Here's how the part is built. I have some questions about the finished solid (model axes, mm). Face numbers are marked on the shaded views. A direction names the side the tool comes from. Round coordinates to 2 decimals unless told otherwise and drop trailing zeros. Write each loop counter-clockwise with the first axis right and the second up, starting at its lowest first coordinate (ties: lowest second). Pieces come first, ordered by that corner, then holes. Notation, with made-up numbers: (89.5, -2.75) -> (138.5, -2.75) arc R23 cw to (138.5, 6.25) -> close; hole circle Ø6 at (44.25, 84). An arc over 180 degrees is marked (long way). Answer in a Markdown table with one row per item.
from build123d import *

# Parameters (mm, degrees)
SKETCH_3_R                       = 7.9
EXTRUDE_1_DEPTH                  = 11.8
FILLET_1_R                       = 6.2
FILLET_2_R                       = 3
CHAMFER_1_SIZE                   = 1
HOLE_WIZARD_4_7_4_7_2_D          = 4.7
SKETCH_18_W                      = 4.7
SKETCH_18_H                      = 8.206022117
HOLE_WIZARD_9_4_9_4_1_AT_2_COUNT = 2
HOLE_WIZARD_9_4_9_4_1_AT_2_PITCH = 30
HOLE_WIZARD_M3_2_D               = 2.5
HOLE_WIZARD_M3_2_DEPTH           = 3
HOLE_WIZARD_M3_2_TIP             = 0.751075774


with BuildPart() as part:
    # 스케치3 → 보스-돌출1 (new body)
    with BuildSketch(Plane.XY):
        with BuildLine():
            Line((-7.45, 0), (7.45, 0))
            Line((7.45, 0), (7.45, 2))
            Line((7.45, 2), (20.6, 2))
            Line((20.6, 2), (20.6, 14.5))
            Line((20.6, 14.5), (9.765842668, 14.5))
            ThreePointArc((9.765842668, 14.5), (0, 22.006022117), (-9.765842668, 14.5))
            Line((-9.765842668, 14.5), (-20.6, 14.5))
            Line((-20.6, 14.5), (-20.6, 2))
            Line((-20.6, 2), (-7.45, 2))
            Line((-7.45, 2), (-7.45, 0))
        make_face()
        with Locations((0, 11.9)):
            Circle(SKETCH_3_R, mode=Mode.SUBTRACT)
    extrude(amount=EXTRUDE_1_DEPTH)

    # 필렛1
    fillet_1_edges = [part.edges().sort_by_distance(p)[0] for p in [
        (-9.765842668, 14.5, 5.9),
        (9.765842668, 14.5, 5.9),
    ]]
    fillet(fillet_1_edges, radius=FILLET_1_R)

    # 필렛2
    fillet_2_edges = [part.edges().sort_by_distance(p)[0] for p in [
        (20.6, 8.25, 0),
        (20.6, 8.25, 11.8),
        (-20.6, 8.25, 11.8),
        (-20.6, 8.25, 0),
    ]]
    fillet(fillet_2_edges, radius=FILLET_2_R)

    # 모따기1
    chamfer_1_edges = [part.edges().sort_by_distance(p)[0] for p in [
        (-7.9, 11.9, 0),
    ]]
    chamfer(chamfer_1_edges, length=CHAMFER_1_SIZE)

    # Ø4.7 (4.7) 지름 구멍2 (through all)
    with Locations(Plane.XZ):
        with Locations((15, 5.9), (-15, 5.9)):
            Hole(HOLE_WIZARD_4_7_4_7_2_D / 2)

    # 스케치18 → Ø9.4 (9.4) 지름 구멍1 (revolve, cut)
    with BuildSketch(Plane(origin=(-15, 13.8, 5.9), x_dir=(0, 0, -1), z_dir=(1, 0, 0))):
        with Locations((2.35, 4.103011058)):
            Rectangle(SKETCH_18_W, SKETCH_18_H)
    hole_wizard_9_4_9_4_1 = revolve(axis=Axis((-15, 7.45, 5.9), (0, 1, 0)), mode=Mode.SUBTRACT)

    # Ø9.4 (9.4) 지름 구멍1 at 2: Ø9.4 (9.4) 지름 구멍1 ×2
    with Locations(*[(i * HOLE_WIZARD_9_4_9_4_1_AT_2_PITCH, 0, 0) for i in range(1, HOLE_WIZARD_9_4_9_4_1_AT_2_COUNT)]):
        add(hole_wizard_9_4_9_4_1, mode=Mode.SUBTRACT)

    # M3 나사 구멍2
    with Locations(Plane.XY.offset(11.8)):
        with Locations((-10, 9.1)):
            Hole(HOLE_WIZARD_M3_2_D / 2, depth=HOLE_WIZARD_M3_2_DEPTH)
            with Locations((0, 0, -(HOLE_WIZARD_M3_2_DEPTH + HOLE_WIZARD_M3_2_TIP / 2))):  # 118° drill point
                Cone(0, HOLE_WIZARD_M3_2_D / 2, HOLE_WIZARD_M3_2_TIP, mode=Mode.SUBTRACT)


solid = part.part
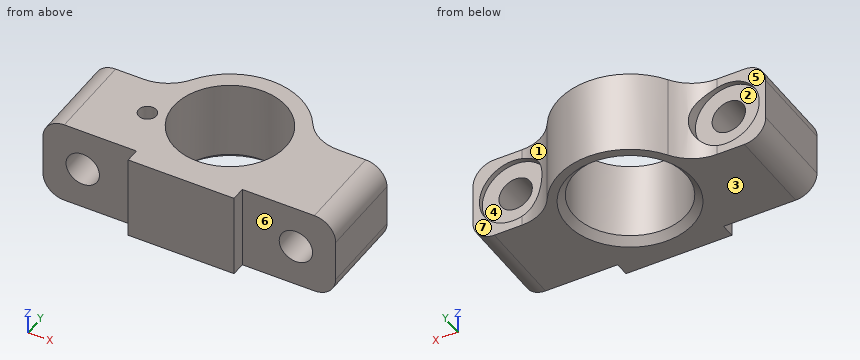
1) I want a section at B-B, the plane x = -15. List the corners of the cut face in (y, z) for me, and give its area (3 significant figures).
Response:
| item | result |
|---|---|
| outline | (2, 0) -> (14.5, 0) -> (14.5, 1.2) -> (13.8, 1.2) -> (13.8, 3.55) -> (2, 3.55) -> close; (2, 8.25) -> (13.8, 8.25) -> (13.8, 10.6) -> (14.5, 10.6) -> (14.5, 11.8) -> (2, 11.8) -> close |
| area | 85.5 mm^2 |
2) I want a section at D-D, the plane z = 11. List the corners of the cut face in (x, y) for me.
Response:
| item | result |
|---|---|
| outline | (-19.64, 2) -> (-7.45, 2) -> (-7.45, 0) -> (7.45, 0) -> (7.45, 2) -> (19.64, 2) -> (19.64, 14.5) -> (13.73, 14.5) arc R6.2 cw to (8.51, 17.35) arc R10.11 ccw to (-8.51, 17.35) arc R6.2 cw to (-13.73, 14.5) -> (-19.64, 14.5) -> close; hole circle Ø2.5 at (-10, 9.1); hole circle Ø15.8 at (0, 11.9) |
3) For pin 1 (2 mm diameter, centred on x = 16, z = 4.5, fed in from +Y); pin 2 (1 mm diameter, centred on y = 1, z = 3, fed in from +X); pin 3 (12.5 mm diameter, centred on x = 0, y = 11.9, fed in from +Z); pin 4 (12 mm diameter, centred on x = 4.5, y = 7, fed in from +Z), each with a flat end and sliding along its axis, tell me the tip position at first contact or that it passes through.
Response:
| item | result |
|---|---|
| pin 1 | stops at y = 13.8 |
| pin 2 | stops at x = 7.45 |
| pin 3 | passes through |
| pin 4 | stops at z = 11.8 |
4) Which directions (+Z, -Z, +X, -X, +Y, -Y) give clear straight access to the entire face, cutting with the end or side of a thin tool? Please do the marked faces 4, 5, 6 and 7.
Response:
| item | result |
|---|---|
| face 4 | +Y |
| face 5 | +Z, -Z, -X, +Y |
| face 6 | +Z, -Z, +X, -Y |
| face 7 | +Z, -Z, +X, +Y |
5) I want a section at A-A, the plane y = 11.9. List the corners of the cut face in (x, z) for me, and give its area (3 significant figures).
Response:
| item | result |
|---|---|
| outline | (-20.6, 3) arc R3 ccw to (-17.6, 0) -> (-8.9, 0) -> (-7.9, 1) -> (-7.9, 11.8) -> (-17.6, 11.8) arc R3 ccw to (-20.6, 8.8) -> close; (7.9, 1) -> (8.9, 0) -> (17.6, 0) arc R3 ccw to (20.6, 3) -> (20.6, 8.8) arc R3 ccw to (17.6, 11.8) -> (7.9, 11.8) -> close; hole circle Ø4.7 at (-15, 5.9); hole circle Ø4.7 at (15, 5.9) |
| area | 256 mm^2 |
6) I need wall thicknesses on line 1 (Y direction, x = 0, z = 5); line 2 (X direction, y = 10.5, z = 6.25); line 3 (Z direction, x = -15, y = 9.75). Which ranges of each line are inside material? Lowest first, please. Write a range as [from, to].
Response:
| item | result |
|---|---|
| line 1 | y = [0, 4], [19.8, 22.01] |
| line 2 | x = [-20.6, -17.32], [-12.68, -7.77], [7.77, 12.68], [17.32, 20.6] |
| line 3 | z = [0, 3.55], [8.25, 11.8] |
7) I want a section at C-C, the plane z = 7. List the corners of the cut face in (x, y) for me.
Response:
| item | result |
|---|---|
| outline | (-20.6, 2) -> (-17.08, 2) -> (-17.08, 13.8) -> (-19.57, 13.8) -> (-19.57, 14.5) -> (-20.6, 14.5) -> close; (-12.92, 2) -> (-7.45, 2) -> (-7.45, 0) -> (7.45, 0) -> (7.45, 2) -> (12.92, 2) -> (12.92, 13.8) -> (10.43, 13.8) -> (10.43, 15.45) arc R6.2 cw to (8.51, 17.35) arc R10.11 ccw to (-8.51, 17.35) arc R6.2 cw to (-10.43, 15.45) -> (-10.43, 13.8) -> (-12.92, 13.8) -> close; (17.08, 2) -> (20.6, 2) -> (20.6, 14.5) -> (19.57, 14.5) -> (19.57, 13.8) -> (17.08, 13.8) -> close; hole circle Ø15.8 at (0, 11.9) |
8) We'd pull the mould along X, two halves only. Please class the marked faces 1, 2 and 3: +X half, -X half, draft (parallel to the pull), parting line (faces both ways), or undercut.
Response:
| item | result |
|---|---|
| face 1 | +X half |
| face 2 | undercut |
| face 3 | draft |
